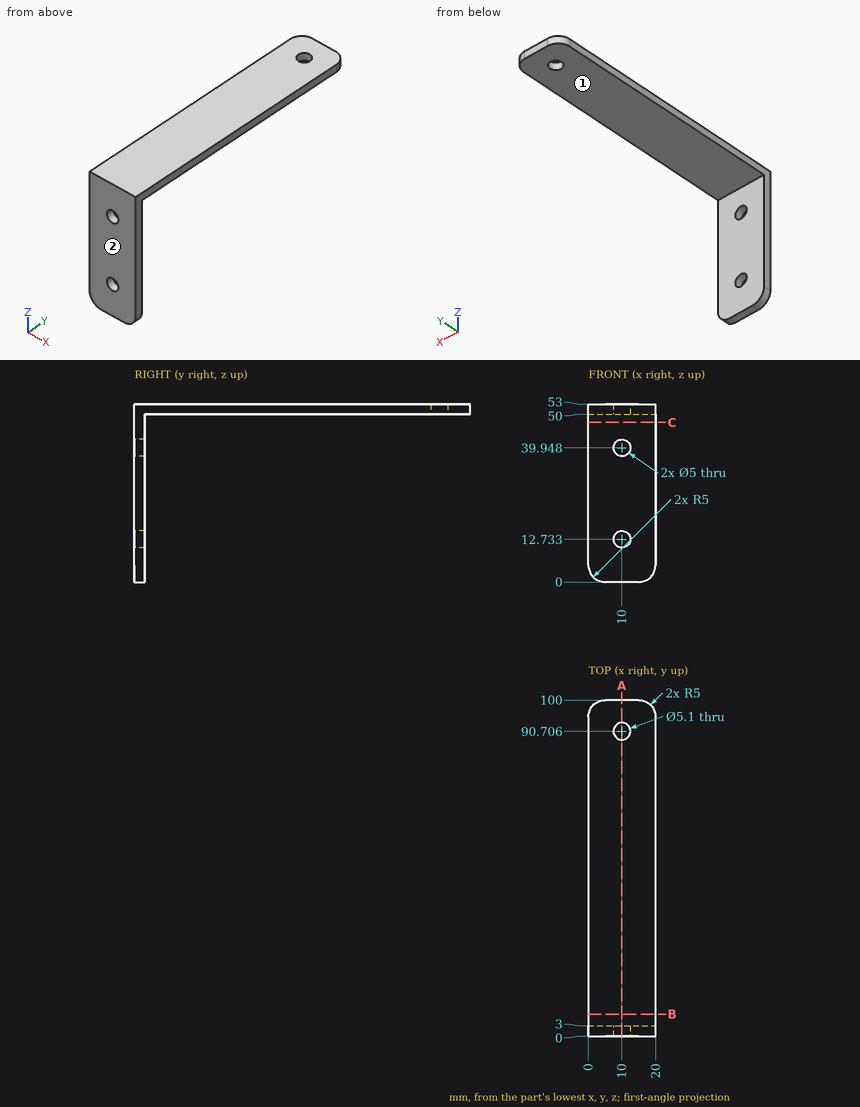
Could you check a few things on this drawing? It's one solid part, dimensions in mm from its lowest x, y, z. A direction names the side the tool comes from. Give positions to 0.01 mm unless a question says otherwise; leave off trailing zeros. Write each loop counter-clockwise with the first axis right and the second up, starting at its lowest first coordinate (ties: lowest second). Pieces come first, ordered by that corner, then holes.
(1) If I drill on L1, parallel to Z at x = 10, y = 1.05; L2, parallel to Y at x = 10, z = 51.1; L3, parallel to Z at x = 16.25, y = 50.5, over which ranges is the centre line in solid material (lowest first)?
Output values:
L1: z = 0 to 10.23, 15.23 to 37.45, 42.45 to 53
L2: y = 0 to 88.16, 93.26 to 100
L3: z = 50 to 53
(2) Will these pins go through, and if not, where does the flat tip stop? pin 1 (6 mm diameter, centred on x = 5.5, y = 39, fed in from -Z); pin 2 (12 mm diameter, centred on x = 2.5, z = 6, fed in from +Y).
Output values:
pin 1: stops at z = 50
pin 2: stops at y = 3
(3) Imagine slicing it at A-A, the plane x = 10. Write out the boundary of the cut face in (y, z).
Output values:
outline: (0, 0) - (3, 0) - (3, 10.23) - (0, 10.23) - close; (0, 15.23) - (3, 15.23) - (3, 37.45) - (0, 37.45) - close; (0, 42.45) - (3, 42.45) - (3, 50) - (88.16, 50) - (88.16, 53) - (0, 53) - close; (93.26, 50) - (100, 50) - (100, 53) - (93.26, 53) - close
(4) On a 3-axis mill with a long thin cutter (end or side, diameter ignored), from which of +Z, -Z, +X, -X, +Y, -Y can I reach the whole of each face in a straight line? I mean the marked faces 1 and 2. Say none if no direction works.
Output values:
face 1: -Z, +X, -X, +Y
face 2: +Z, -Z, +X, -X, -Y
(5) Imagine slicing it at B-B, the plane y = 6.5. Write out the boundary of the cut face in (x, z), and give its area (3 significant figures).
Output values:
outline: (0, 50) - (20, 50) - (20, 53) - (0, 53) - close
area: 60.0 mm2
(6) Imagine slicing it at C-C, the plane z = 47.5. Write out the boundary of the cut face in (x, y), and give its area (3 significant figures).
Output values:
outline: (0, 0) - (20, 0) - (20, 3) - (0, 3) - close
area: 60.0 mm2
